```python
from build123d import *

# Parameters (mm, degrees)
F0_W     = 152.4
F0_H     = 76.2
F1_DEPTH = 12.7
F2_R     = 9.525
F3_DEPTH = 12.701


with BuildPart() as f1:
    # F0 (on Front) → F1 (new body)
    with BuildSketch(Plane.XZ):
        Rectangle(F0_W, F0_H)
    extrude(amount=F1_DEPTH)

    # F2 (on face) → F3 (cut, through all)
    with BuildSketch(Plane(origin=(0, 0, 0), x_dir=(-1, 0, 0), z_dir=(0, 1, 0))):
        with Locations((63.5, 25.4)):
            Circle(F2_R)
        with Locations((63.5, -25.4)):
            Circle(F2_R)
        with Locations((-63.5, -25.4)):
            Circle(F2_R)
        with Locations((-63.5, 25.4)):
            Circle(F2_R)
    extrude(amount=-F3_DEPTH, mode=Mode.SUBTRACT)

    # F4 (on Top) → F5 (revolve)
    with BuildSketch(Plane.XY):
        with BuildLine():
            ThreePointArc((-20.746347, 0), (-20.507447, -0.003656), (-20.268548, 0))
            Line((-20.268548, 0), (-20.746347, 0))
        make_face()
        Polygon((-12.7, 0), (0, 0), (0, 38.1), (-12.7, 38.1), (-12.7, 7.803791), align=None)
        with BuildLine():
            Line((-20.268548, 0), (-12.7, 0))
            Line((-12.7, 0), (-12.7, 7.803791))
            ThreePointArc((-12.7, 7.803791), (-14.902921, 2.368212), (-20.268548, 0))
        make_face()
    revolve(axis=Axis((0, 19.05, 0), (0, 1, 0)))

    # F6 (on Top) → F7 (revolve, cut)
    with BuildSketch(Plane.XY):
        with BuildLine():
            Line((-15.973667, 12.416507), (-7.864556, 12.416507))
            ThreePointArc((-7.864556, 12.416507), (-6.068504, 13.160456), (-5.324556, 14.956507))
            Line((-5.324556, 14.956507), (-5.324556, 17.437313))
            ThreePointArc((-5.324556, 17.437313), (-6.068504, 19.233365), (-7.864556, 19.977313))
            Line((-7.864556, 19.977313), (-15.973667, 19.977313))
            Line((-15.973667, 19.977313), (-15.973667, 12.416507))
        make_face()
    revolve(axis=Axis((0, 8.098455, 0), (0, 1, 0)), mode=Mode.SUBTRACT)


solid = f1.part
```
Verification items for the finished model (mm, model axes). A direction names the side the tool comes from. Give positions to 0.01 mm unless a question says otherwise; leave off trailing zeros. Loops run counter-clockwise (first coordinate to the right, second up) from the corner with the lowest first, then second, coordinate; pieces in that order, holes last.
1. Section check D-D, the plane x = 25.5. Enter the section's corners in (y, z).
2. Mould release check, pull along Y, two halves, no side actions. Record for faces 4 (the flat face through (0, 38.1, 0)), 5 (the flat face through (-0.2, 19.977, -8.3)), 6 (the cylindrical face through (54.7, -6.26, 21.75)): released by +Y, released by -Y, zero draft, split by the parting line, or undercut.
3. Section check C-C, the plane x = -63.5. Enter the section's corners in (y, z) (3 decimals).
4. Section check A-A, the plane z = 25.4. Enter the section's corners in (x, y) (3 decimals), then the cut area to 3 significant figures.
5. Set-up check for faces 1 (the flat face through (0.2, 12.417, -8.3)), 2 (the flat face through (-18, 0, 17)), 3 (the flat face through (-1, -6, 38.1)): record each of +Z, -Z, +X, -X, +Y, -Y from which the full face is reachable in a straight line by a thin tool's end or side.
6. Section check B-B, the plane y = -5. Enter the section's corners in (x, z) (3 decimals).
7. Thickness scan on line 1 (Z direction, x = 63.5, y = -9) (3 decimals); line 2 (X direction, y = -1, z = -32); line 3 (X direction, y = -10, z = 18). Record the ranges inside material, lowest first.
8. Go/stop test with flat-tipped pins: pin 1 Ø10 at (x, z) = (57, -19.5) entering from +Y; pin 2 Ø2 at (y, z) = (24, 0.5) entering from -X. Record where each tip stops, or that it passes through.
Geometry says:
1. outline: (-12.7, -38.1) - (0, -38.1) - (0, 38.1) - (-12.7, 38.1) - close
2. face 4: released by +Y
2. face 5: undercut
2. face 6: zero draft
3. outline: (-12.7, -38.1) - (0, -38.1) - (0, -34.925) - (-12.7, -34.925) - close; (-12.7, -15.875) - (0, -15.875) - (0, 15.875) - (-12.7, 15.875) - close; (-12.7, 34.925) - (0, 34.925) - (0, 38.1) - (-12.7, 38.1) - close
4. outline: (-76.2, -12.7) - (-73.025, -12.7) - (-73.025, 0) - (-76.2, 0) - close; (-53.975, -12.7) - (53.975, -12.7) - (53.975, 0) - (-53.975, 0) - close; (73.025, -12.7) - (76.2, -12.7) - (76.2, 0) - (73.025, 0) - close
4. area: 1,450 mm2
5. face 1: none
5. face 2: +Y
5. face 3: +Z, +X, -X, +Y, -Y
6. outline: (-76.2, -38.1) - (76.2, -38.1) - (76.2, 38.1) - (-76.2, 38.1) - close; hole circle Ø19.05 at (-63.5, -25.4); hole circle Ø19.05 at (-63.5, 25.4); hole circle Ø19.05 at (63.5, -25.4); hole circle Ø19.05 at (63.5, 25.4)
7. line 1: z = -38.1 to -34.925, -15.875 to 15.875, 34.925 to 38.1
7. line 2: x = -76.2 to -70.37, -56.63 to 56.63, 70.37 to 76.2
7. line 3: x = -76.2 to -69.5, -57.5 to 57.5, 69.5 to 76.2
8. pin 1: stops at y = 0
8. pin 2: stops at x = -12.7
